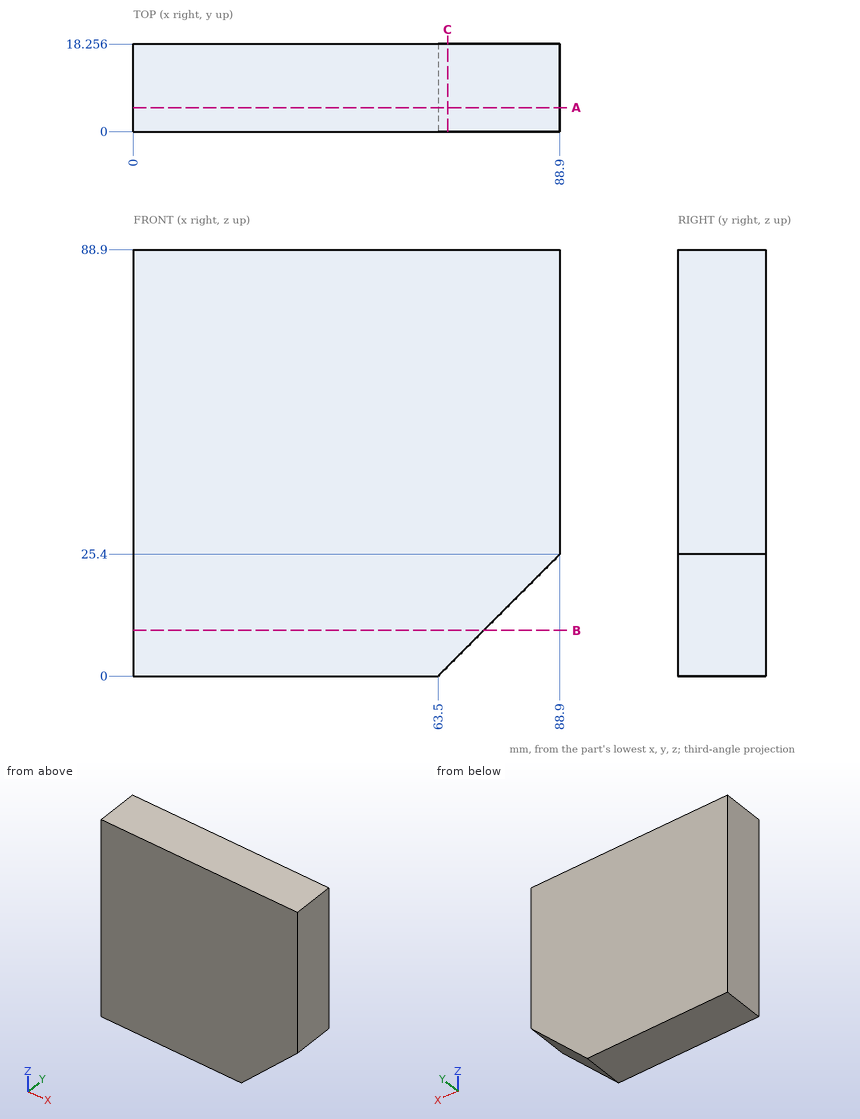
The drawing under review shows one solid part. Ordinate dimensions are in mm from its lowest x, y, z. Round coordinates to 2 decimals unless told otherwise and drop trailing zeros. Order: outer loops, then holes, each group sorted by start corner. A loop starts at its lowest first (then second) coordinate and runs counter-clockwise, first axis right, second up. Notation, with made-up numbers: (83, 58.25) - (114, 58.25) arc R17 cw to (114, 77.25) - close; hole circle Ø10 at (54, 86.25). An arc over 180 degrees is marked (long way). Return JSON: item names as keys, results as strings.
Q1. Consider section C-C on x = 65.5. Write out the cut boundary in (y, z).
Computed values:
{"outline": "(0, 2) - (18.26, 2) - (18.26, 88.9) - (0, 88.9) - close"}
Q2. Consider section A-A on y = 5. Write out the cut boundary in (x, z).
Computed values:
{"outline": "(0, 0) - (63.5, 0) - (88.9, 25.4) - (88.9, 88.9) - (0, 88.9) - close"}
Q3. Wall thickness on L1, parallel to X at y = 5, z = 25; L2, parallel to Z at x = 72, y = 1.75; L3, parallel to Z at x = 75.5, y = 1.25: over which ranges is each line inside the solid? List them lowest first. Write a range as [from, to].
Computed values:
{"L1": "x = [0, 88.5]", "L2": "z = [8.5, 88.9]", "L3": "z = [12, 88.9]"}
Q4. Consider section B-B on z = 9.5. Write out the cut boundary in (x, y).
Computed values:
{"outline": "(0, 0) - (73, 0) - (73, 18.26) - (0, 18.26) - close"}
Q5. For pin 1 Ø2 at (x, y) = (54, 5.5) entering from -Z, flat-tipped, find the tip position at first contact; note if it passes through.
Computed values:
{"pin 1": "stops at z = 0"}
